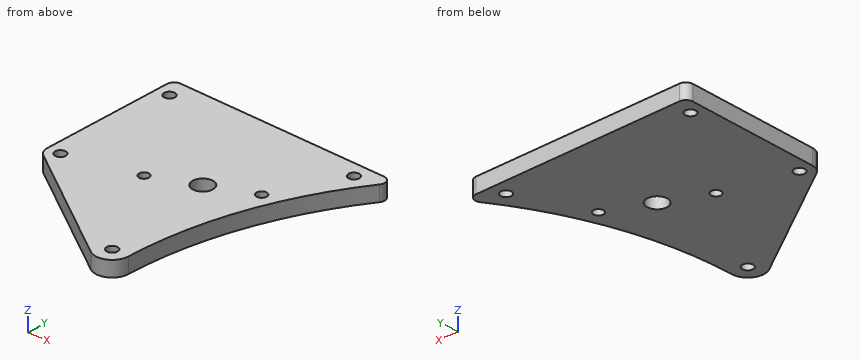
```python
from build123d import *

# Parameters (mm, degrees)
SKETCH1_R           = 2.1
SKETCH1_R_2         = 4.248828393
SKETCH1_R_3         = 2.248
BOSS_EXTRUDE1_DEPTH = 6.35


with BuildPart() as part:
    # Sketch1 → Boss-Extrude1 (new body)
    with BuildSketch(Plane.XY):
        with BuildLine():
            Line((-164.857630571, -5.684506245), (-217.606823936, 30.483431618))
            ThreePointArc((-217.606823936, 30.483431618), (-219.355038804, 32.447489975), (-219.986286008, 35))
            Line((-219.986286008, 35), (-219.986286008, 90.85821565))
            ThreePointArc((-219.986286008, 90.85821565), (-219.086022557, 93.00090238), (-216.925548391, 93.857600744))
            Line((-216.925548391, 93.857600744), (-129.300414508, 92.083189784))
            ThreePointArc((-129.300414508, 92.083189784), (-126.69155089, 90.452464344), (-126.890346887, 87.38229904))
            ThreePointArc((-126.890346887, 87.38229904), (-147.116480921, 45.755517262), (-154.067603079, 0))
            ThreePointArc((-154.067603079, 0), (-157.747437287, -6.09791572), (-164.857630571, -5.684506245))
        make_face()
        with Locations((-185.554258914, 42.046855659)):
            Circle(SKETCH1_R, mode=Mode.SUBTRACT)
        with Locations((-149.938627555, 57.675374206)):
            Circle(SKETCH1_R, mode=Mode.SUBTRACT)
        with Locations((-167.746443234, 49.861114932)):
            Circle(SKETCH1_R_2, mode=Mode.SUBTRACT)
        with Locations((-214.51, 86)):
            Circle(SKETCH1_R_3, mode=Mode.SUBTRACT)
        with Locations((-214.51, 35)):
            Circle(SKETCH1_R_3, mode=Mode.SUBTRACT)
        with Locations((-136.51, 86)):
            Circle(SKETCH1_R_3, mode=Mode.SUBTRACT)
        with Locations((-160.96, 0)):
            Circle(SKETCH1_R_3, mode=Mode.SUBTRACT)
    extrude(amount=BOSS_EXTRUDE1_DEPTH)


solid = part.part
```
Part model, mm, in its own coordinate system. Round coordinates to 2 decimals unless told otherwise and drop trailing zeros. Loops run counter-clockwise (first coordinate to the right, second up) from the corner with the lowest first, then second, coordinate; pieces in that order, holes last.
Item 1: Cut at D-D, the plane z = 3. Give the cut face in (x, y).
Item 2: Drop flat-ended pins along their axis: P1, Ø1, axis at y = 12, z = 5, coming from the -X side; P2, Ø1.5, axis at x = -200.5, z = 4, coming from the +Y side; P3, Ø1.5, axis at x = -208, z = 4, coming from the +Y side; P4, Ø5, axis at x = -149.94, y = 57.68, coming from the +Z side. Give the stop position or say it passes through.
Item 3: Cut at A-A, the plane y = 86. Give the cut face in (x, z), then the cut area to 3 significant figures.
Item 4: Drill centre lines: line 1 (Y direction, x = -214.51, z = 2); line 2 (Y direction, x = -215, z = 1.5); line 3 (X direction, y = 6, z = 3.25). Where is each one in solid material? Low to high.
Item 5: Cut at B-B, the plane x = -136.51. Give the cut face in (y, z).
Item 6: Cut at C-C, the plane y = 53. Give the cut face in (x, z), then the cut area to 3 significant figures.
A:
1. outline: (-219.99, 35) arc R5.48 ccw to (-217.61, 30.48) - (-164.86, -5.68) arc R6.89 ccw to (-154.07, 0) arc R154.07 cw to (-126.89, 87.38) arc R3 ccw to (-129.3, 92.08) - (-216.93, 93.86) arc R3 ccw to (-219.99, 90.86) - close; hole circle Ø4.5 at (-214.51, 35); hole circle Ø4.5 at (-214.51, 86); hole circle Ø4.2 at (-185.55, 42.05); hole circle Ø8.5 at (-167.75, 49.86); hole circle Ø4.5 at (-160.96, 0); hole circle Ø4.2 at (-149.94, 57.68); hole circle Ø4.5 at (-136.51, 86)
2. P1: stops at x = -191.38
2. P2: stops at y = 93.54
2. P3: stops at y = 93.69
2. P4: stops at z = 6.35
3. outline: (-219.99, 0) - (-216.76, 0) - (-216.76, 6.35) - (-219.99, 6.35) - close; (-212.26, 0) - (-138.76, 0) - (-138.76, 6.35) - (-212.26, 6.35) - close; (-134.26, 0) - (-127.83, 0) - (-127.83, 6.35) - (-134.26, 6.35) - close
3. area: 528 mm2
4. line 1: y = 28.36 to 32.75, 37.25 to 83.75, 88.25 to 93.81
4. line 2: y = 28.7 to 32.81, 37.19 to 83.81, 88.19 to 93.82
4. line 3: x = -181.9 to -153.95
5. outline: (71.43, 0) - (83.75, 0) - (83.75, 6.35) - (71.43, 6.35) - close; (88.25, 0) - (92.23, 0) - (92.23, 6.35) - (88.25, 6.35) - close
6. outline: (-219.99, 0) - (-170.61, 0) - (-170.61, 6.35) - (-219.99, 6.35) - close; (-164.88, 0) - (-144.66, 0) - (-144.66, 6.35) - (-164.88, 6.35) - close
6. area: 442 mm2
